For this review, take the finished solid that the model builds, in its own axes (mm). A direction names the side the tool comes from. Give positions to 0.01 mm unless a question says otherwise; leave off trailing zeros. Loops run counter-clockwise (first coordinate to the right, second up) from the corner with the lowest first, then second, coordinate; pieces in that order, holes last. Notation, with made-up numbers: (6.25, 8) - (32.25, 8) arc R22 cw to (32.25, 36) - close; hole circle Ø2 at (20.25, 32). An arc over 180 degrees is marked (long way). Put each result on its own line as item: value. Start each with the question number.
from build123d import *

# Parameters (mm, degrees)
BOSS_EXTRUDE2_DEPTH = 300
FILLET5_R           = 0.5
SKETCH3_R           = 3
CUT_EXTRUDE2_DEPTH  = 4.5
SKETCH4_R           = 1.75
CUT_EXTRUDE3_DEPTH  = 14.5
SKETCH5_W           = 12
SKETCH5_H           = 4.057387372
CUT_EXTRUDE4_DEPTH  = 682.5


with BuildPart() as part:
    # Sketch1 → Boss-Extrude2 (new body)
    with BuildSketch(Plane.XY):
        Polygon((0, 0), (12, 0), (12, 8.403449878), (9.5, 9.846825551), (12, 11.290201224), (12, 12), (0, 12), (0, 11.290201224), (2.5, 9.846825551), (0, 8.403449878), align=None)
    extrude(amount=BOSS_EXTRUDE2_DEPTH)

    # Fillet5
    # the kernel refuses this fillet: 0.5 mm, written as the material it adds along each edge
    with BuildSketch(Plane(origin=(2.5, 9.846825551, 0), x_dir=(-0.8660254037844382, 0.5000000000000009, 0), z_dir=(0, 0, 1)), Plane(origin=(9.5, 9.846825551, 0), x_dir=(0.8660254037844379, -0.5000000000000013, 0), z_dir=(0, 0, 1))) as fillet5_piece_1:
        with BuildLine():
            CenterArc((FILLET5_R * 1.73205080757, FILLET5_R), FILLET5_R, 150, 120)
            Line((FILLET5_R * 0.866025403784, FILLET5_R * 1.5), (0, 0))
            Line((0, 0), (FILLET5_R * 1.73205080757, 0))
        make_face()
    extrude(amount=300)
    # the kernel refuses this fillet: 0.5 mm, written as the material it takes off along each edge
    with BuildSketch(Plane(origin=(0, 8.403449878, -0.721687836), x_dir=(0, -1, 0), z_dir=(0, 0, 1))) as fillet5_2_piece_1:
        with BuildLine():
            CenterArc((FILLET5_R * 0.57735026919, FILLET5_R), FILLET5_R, 210, 60)
            Line((-FILLET5_R * 0.288675134595, FILLET5_R * 0.5), (0, 0))
            Line((0, 0), (FILLET5_R * 0.57735026919, 0))
        make_face()
    extrude(amount=301.443375673, mode=Mode.SUBTRACT)
    with BuildSketch(Plane(origin=(0, 11.290201224, -0.721687836), x_dir=(0, 1, 0), z_dir=(0, 0, 1)), Plane(origin=(12, 11.290201224, -0.721687836), x_dir=(-0.8660254037844355, -0.5000000000000052, 0), z_dir=(0, 0, 1)), Plane(origin=(12, 8.403449878, -0.721687836), x_dir=(0, -1, 0), z_dir=(0, 0, 1))) as fillet5_2_piece_2:
        with BuildLine():
            CenterArc((FILLET5_R * 0.57735026919, -FILLET5_R), FILLET5_R, 90, 60)
            Line((-FILLET5_R * 0.288675134595, -FILLET5_R * 0.5), (0, 0))
            Line((0, 0), (FILLET5_R * 0.57735026919, 0))
        make_face()
    extrude(amount=301.443375673, mode=Mode.SUBTRACT)
    with BuildSketch(Plane(origin=(0, 12, -1.25), x_dir=(1, 0, 0), z_dir=(0, 0, 1)), Plane(origin=(12, 12, -1.25), x_dir=(0, -1, 0), z_dir=(0, 0, 1))) as fillet5_2_piece_3:
        with BuildLine():
            CenterArc((FILLET5_R, -FILLET5_R), FILLET5_R, 90, 90)
            Line((0, -FILLET5_R), (0, 0))
            Line((0, 0), (FILLET5_R, 0))
        make_face()
    extrude(amount=302.5, mode=Mode.SUBTRACT)

    # Sketch3 → Cut-Extrude2 (cut)
    with BuildSketch(Plane(origin=(0, 12, 0), x_dir=(1, 0, 0), z_dir=(0, 1, 0))):
        with Locations((6, -490)):
            Circle(SKETCH3_R)
        with Locations((6, -440)):
            Circle(SKETCH3_R)
        with Locations((6, -415)):
            Circle(SKETCH3_R)
        with Locations((6, -390)):
            Circle(SKETCH3_R)
        with Locations((6, -365)):
            Circle(SKETCH3_R)
        with Locations((6, -340)):
            Circle(SKETCH3_R)
        with Locations((6, -315)):
            Circle(SKETCH3_R)
        with Locations(Location((6, -290, 0), (0, 0, 180))):
            Circle(SKETCH3_R)
        with Locations(Location((6, -265, 0), (0, 0, 180))):
            Circle(SKETCH3_R)
        with Locations(Location((6, -240, 0), (0, 0, 180))):
            Circle(SKETCH3_R)
        with Locations(Location((6, -215, 0), (0, 0, 180))):
            Circle(SKETCH3_R)
        with Locations(Location((6, -190, 0), (0, 0, 180))):
            Circle(SKETCH3_R)
        with Locations(Location((6, -165, 0), (0, 0, 180))):
            Circle(SKETCH3_R)
        with Locations(Location((6, -140, 0), (0, 0, 180))):
            Circle(SKETCH3_R)
        with Locations(Location((6, -115, 0), (0, 0, 180))):
            Circle(SKETCH3_R)
        with Locations(Location((6, -90, 0), (0, 0, 180))):
            Circle(SKETCH3_R)
        with Locations(Location((6, -65, 0), (0, 0, 180))):
            Circle(SKETCH3_R)
        with Locations(Location((6, -40, 0), (0, 0, 180))):
            Circle(SKETCH3_R)
        with Locations(Location((6, -15, 0), (0, 0, 180))):
            Circle(SKETCH3_R)
        with Locations((6, -465)):
            Circle(SKETCH3_R)
    extrude(amount=-CUT_EXTRUDE2_DEPTH, mode=Mode.SUBTRACT)

    # Sketch4 → Cut-Extrude3 (cut)
    with BuildSketch(Plane(origin=(0, 12, 0), x_dir=(1, 0, 0), z_dir=(0, 1, 0))):
        with Locations(Location((6, -15, 0), (0, 0, 180))):
            Circle(SKETCH4_R)
        with Locations(Location((6, -40, 0), (0, 0, 180))):
            Circle(SKETCH4_R)
        with Locations(Location((6, -65, 0), (0, 0, 180))):
            Circle(SKETCH4_R)
        with Locations(Location((6, -90, 0), (0, 0, 180))):
            Circle(SKETCH4_R)
        with Locations(Location((6, -115, 0), (0, 0, 180))):
            Circle(SKETCH4_R)
        with Locations(Location((6, -140, 0), (0, 0, 180))):
            Circle(SKETCH4_R)
        with Locations(Location((6, -165, 0), (0, 0, 180))):
            Circle(SKETCH4_R)
        with Locations(Location((6, -190, 0), (0, 0, 180))):
            Circle(SKETCH4_R)
        with Locations(Location((6, -215, 0), (0, 0, 180))):
            Circle(SKETCH4_R)
        with Locations(Location((6, -240, 0), (0, 0, 180))):
            Circle(SKETCH4_R)
        with Locations(Location((6, -265, 0), (0, 0, 180))):
            Circle(SKETCH4_R)
        with Locations(Location((6, -290, 0), (0, 0, 180))):
            Circle(SKETCH4_R)
        with Locations((6, -315)):
            Circle(SKETCH4_R)
        with Locations((6, -340)):
            Circle(SKETCH4_R)
        with Locations((6, -365)):
            Circle(SKETCH4_R)
        with Locations((6, -390)):
            Circle(SKETCH4_R)
        with Locations((6, -415)):
            Circle(SKETCH4_R)
        with Locations((6, -440)):
            Circle(SKETCH4_R)
        with Locations((6, -465)):
            Circle(SKETCH4_R)
        with Locations((6, -490)):
            Circle(SKETCH4_R)
    extrude(amount=-CUT_EXTRUDE3_DEPTH, mode=Mode.SUBTRACT)

    # Sketch5 → Cut-Extrude4 (cut)
    with BuildSketch(Plane(origin=(0, 0, 0), x_dir=(-1, 0, 0), z_dir=(0, 0, -1))):
        with Locations((-6, 2.028693686)):
            Rectangle(SKETCH5_W, SKETCH5_H)
    extrude(amount=-CUT_EXTRUDE4_DEPTH, mode=Mode.SUBTRACT)


solid = part.part
1) Take a section at A-A on y = 5.5. State how many separate pieces and enclosed holes the cut face has, and give its area (3 significant figures).
2) Take a section at B-B on z = 228. State the section outline as (x, y) points.
3) Machinability: for faces 1 (the flat face through (6, 8, 300)), 2 (the flat face through (4, 7.5, 65)), which of the approach directions +Z, -Z, +X, -X, +Y, -Y give a long, thin tool a straight path to every point of the face, cutting with its end or side? Answer none if there is none.
4) Wall thickness on probe 1 along X at (y, z) = (5.5, 65); probe 2 along X at (y, z) = (11.5, 38); probe 3 along X at (y, z) = (11.5, 278.5): over which ranges is each line inside the solid? List them lowest first.
5) Insertion check: P1, Ø1, axis at y = 7, z = 239, coming from the -X side; P2, Ø3, axis at x = 6.5, z = 164, coming from the +Y side. Each pin has a flat end and moves straight along its axis. Give the tip position at first contact, or say it passes through.
6) Mouldability with a two-part tool opening along X and no side actions: class faces 3 (the flat face through (6, 12, 148)), 4 (the cylindrical face through (6, 10, 43)) as released by +X, released by -X, zero draft, split by the parting line, or undercut.
Answers follow:
1. separate pieces: 1
1. enclosed holes: 12
1. area: 3,480 mm2
2. outline: (0, 4.06) - (12, 4.06) - (12, 8.11) arc R0.5 ccw to (11.75, 8.55) - (10.25, 9.41) arc R0.5 cw to (10.25, 10.28) - (11.75, 11.15) arc R0.5 ccw to (12, 11.54) arc R0.5 ccw to (11.5, 12) - (0.5, 12) arc R0.5 ccw to (0, 11.54) arc R0.5 ccw to (0.25, 11.15) - (1.75, 10.28) arc R0.5 cw to (1.75, 9.41) - (0.25, 8.55) arc R0.5 ccw to (0, 8.11) - close
3. face 1: +Z, +X, -X, +Y, -Y
3. face 2: +Y
4. probe 1: 0 to 4.25, 7.75 to 12
4. probe 2: 0.01 to 3.76, 8.24 to 11.99
4. probe 3: 0.01 to 11.99
5. P1: x = 0
5. P2: y = 7.5
6. face 3: zero draft
6. face 4: undercut
